Verification items for the finished model (mm, model axes). Face numbers are marked on the shaded views. A direction names the side the tool comes from. Round coordinates to 2 decimals unless told otherwise and drop trailing zeros. Order: outer loops, then holes, each group sorted by start corner. A loop starts at its lowest first (then second) coordinate and runs counter-clockwise, first axis right, second up. Notation, with made-up numbers: (76, 84) -> (131, 84) arc R30 ccw to (131, 107) -> close; hole circle Ø5 at (15.25, 9). An arc over 180 degrees is marked (long way). Put each result on its own line as item: value.
from build123d import *

# Parameters (mm, degrees)
F0_R     = 5.1181
F1_DEPTH = 3.556
F2_R     = 4.0767
F3_DEPTH = 1.016
F4_R     = 1.533026
F5_W     = 1.221381
F5_H     = 1.078277
F6_DEPTH = 5.4864


with BuildPart() as f1:
    # F0 (on Top) → F1 (new body)
    with BuildSketch(Plane.XY):
        Circle(F0_R)
    extrude(amount=F1_DEPTH)

    # F2 (on Top) → F3 (cut)
    with BuildSketch(Plane.XY):
        Circle(F2_R)
    extrude(amount=F3_DEPTH, mode=Mode.SUBTRACT)

    # F4
    f4_edges = [f1.edges().sort_by_distance(p)[0] for p in [
        (-5.1181, 0, 3.556),
    ]]
    fillet(f4_edges, radius=F4_R)

    # F5 (on Front) → F6 (cut)
    with BuildSketch(Plane.XZ):
        with Locations((-0.060498, 1.36471)):
            Rectangle(F5_W, F5_H)
    extrude(amount=F6_DEPTH, mode=Mode.SUBTRACT)


solid = f1.part
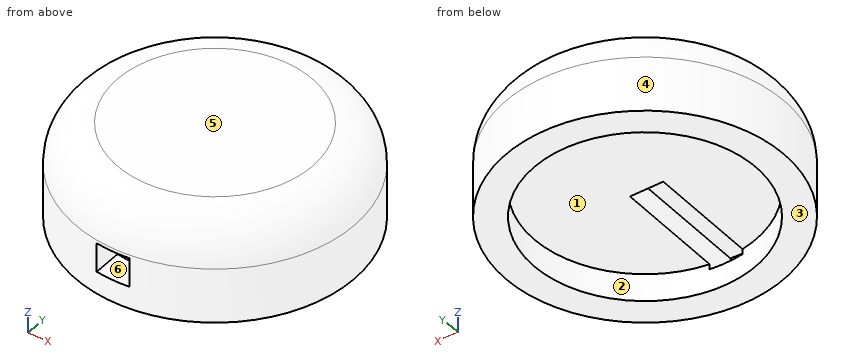
Item 1: Section check B-B on z = 1.15. Record the boundary of the cut face in (x, y).
Check sheet entries:
outline: (-0.67, -5.07) -> (-0.67, 0) -> (0.55, 0) -> (0.55, -5.09) arc R5.12 ccw (long way) to start
Item 2: Gauge pin test, flat ends, axial feed: pin 1 Ø0.9 at (y, z) = (-1.5, 1.5) entering from -X; pin 2 Ø1 at (y, z) = (-3.5, 1.5) entering from +X; pin 3 Ø2 at (x, z) = (2, 3) entering from -Y; pin 4 Ø3 at (x, y) = (3, 2.5) entering from -Z. Record the tip position at first contact, or that the pin passes through.
Check sheet entries:
pin 1: stops at x = -5.01
pin 2: stops at x = 4.15
pin 3: stops at y = -4.93
pin 4: stops at z = 0
Item 3: Section check A-A on x = 0. Record the boundary of the cut face in (y, z).
Check sheet entries:
outline: (-5.12, 0) -> (-4.08, 0) -> (-4.08, 0.83) -> (-5.12, 0.83) -> close; (-5.12, 1.9) -> (0, 1.9) -> (0, 1.02) -> (4.08, 1.02) -> (4.08, 0) -> (5.12, 0) -> (5.12, 2.02) arc R1.53 ccw to (3.59, 3.56) -> (-3.59, 3.56) arc R1.53 ccw to (-5.12, 2.02) -> close
Item 4: Section check C-C on z = 2.45. Record the boundary of the cut face in (x, y).
Check sheet entries:
outline: circle Ø10.11 at (0, 0)
Item 5: Release check for a two-part mould opening along Y. For the marked faces 1, 2, 3 and 4 record: +Y half, -Y half, draft (parallel to the pull), parting line (faces both ways), or undercut.
Check sheet entries:
face 1: undercut
face 2: undercut
face 3: draft
face 4: parting line
Item 6: Material ranges on L1, parallel to Y at x = 0, z = 0.55; L2, parallel to Z at x = -3.25, y = -0.75; L3, parallel to X at y = -2, z = 1.8, recorded low to high. Write a range as [from, to].
Check sheet entries:
L1: y = [-5.12, -4.08], [4.08, 5.12]
L2: z = [1.02, 3.56]
L3: x = [-4.71, -0.67], [0.55, 4.71]
Item 7: Tool access check on the marked faces 5 and 6. Record the directions out of +Z, -Z, +X, -X, +Y, -Y that give a thin tool (end or side, any length) a straight path to the whole face; none if there is none.
Check sheet entries:
face 5: +Z, +X, -X, +Y, -Y
face 6: -Y
